Work out the finished part from the listing and answer in its coordinate system (mm). A direction names the side the tool comes from. Coordinates: 2 decimals unless noted, no trailing zeros. Order: outer loops, then holes, each group sorted by start corner. A loop starts at its lowest first (then second) coordinate and runs counter-clockwise, first axis right, second up. Notation, with made-up numbers: (-5.5, -26) -> (22.5, -26) arc R16 cw to (22.5, -8) -> close; hole circle Ø4 at (52.25, -15). An arc over 180 degrees is marked (long way). Write item = value, one per line. Start each with the question number.
Q1. The part is cut by section C-C, the plane y = -8. Determine the outline of the cut face in (x, z), plus the area to 3 significant figures.
Q2. Which of the six approach directions +Z, -Z, +X, -X, +Y, -Y give full straight-line access (tool end or side, diameter ignored) to faces 4 (the flat face through (4, -6, -120)), 5 (the flat face through (3.94, -8.17, 24.15)), 6 (the flat face through (-19, -22, -61))?
Q3. The part is cut by section B-B, the plane x = 2. Determine the outline of the cut face in (y, z), plus the area to 3 significant figures.
Q4. The part is cut by section D-D, the plane z = 22. Determine the outline of the cut face in (x, y), plus the area to 3 significant figures.
Q5. Flat-ended cylindrical pins translate along their axes: pin 1 (1.6 mm diameter, centred on x = -43, y = -13.5, fed in from -Z); pin 2 (1.5 mm diameter, centred on x = -34.5, z = -126, fed in from +Y); pin 3 (8 mm diameter, centred on y = -7, z = -4.5, fed in from +X); pin 4 (1.6 mm diameter, centred on x = -40.5, y = -14, fed in from +Z). Find the tip coordinate at first contact, or state that the pin passes through.
Q6. For a pull along X with two mould halves and no side action, classify faces 1 (the flat face through (-42, -13, -111)), 2 (the flat face through (-38, -16, -59)), 3 (the flat face through (-46, -16, -59)) as +X half, -X half, draft (parallel to the pull), parting line (faces both ways), or undercut.
Q7. The part is cut by section A-A, the plane z = -45. Determine the outline of the cut face in (x, y), plus the area to 3 significant figures.
Q8. Straight lines are drawn through the part: L1, parallel to X at y = -17, z = 8; L2, parallel to Z at x = -14, y = -27; L3, parallel to X at y = -25.25, z = 22. For each, find the intervals that lie inside material, in ascending order. Write a range as from..to.
```python
from build123d import *

# Parameters (mm, degrees)
DODANIE_WYCI_GNI_CIE1_DEPTH = 8
DODANIE_WYCI_GNI_CIE2_REACH = 171.163
SZKIC2_W                    = 200
SZKIC2_H                    = 8
ZAOKR_GLENIE1_R             = 3
ZAOKR_GLENIE2_R             = 3
SZKIC3_R                    = 7.5
WYTNIJ_WYCI_GNI_CIE1_DEPTH  = 170.162643752


with BuildPart() as part:
    # Szkic1 → Dodanie-wyci_gni_cie1 (new body)
    with BuildSketch(Plane(origin=(0, 0, 0), x_dir=(0, 0, -1), z_dir=(1, 0, 0))):
        with BuildLine():
            Line((0, 0), (-8.660254038, 0))
            ThreePointArc((-8.660254038, 0), (-9.954349263, -0.170370869), (-11.160254038, -0.669872981))
            Line((-11.160254038, -0.669872981), (-37.5, -15.877132403))
            ThreePointArc((-37.5, -15.877132403), (-39.330127019, -17.707259422), (-40, -20.207259422))
            Line((-40, -20.207259422), (-40, -30))
            Line((-40, -30), (160, -30))
            Line((160, -30), (160, -20.207259422))
            ThreePointArc((160, -20.207259422), (159.330127019, -17.707259422), (157.5, -15.877132403))
            Line((157.5, -15.877132403), (131.160254038, -0.669872981))
            ThreePointArc((131.160254038, -0.669872981), (129.954349263, -0.170370869), (128.660254038, 0))
            Line((128.660254038, 0), (120, 0))
            Line((120, 0), (120, -13))
            Line((120, -13), (102.3, -13))
            Line((102.3, -13), (102.3, -15))
            Line((102.3, -15), (17.7, -15))
            Line((17.7, -15), (17.7, -13))
            Line((17.7, -13), (0, -13))
            Line((0, -13), (0, 0))
        make_face()
    extrude(amount=DODANIE_WYCI_GNI_CIE1_DEPTH)


with BuildPart() as body_2:
    # Lustro3: mirrored copy
    add(part.part.mirror(Plane.ZY.offset(19)))

    # Szkic2 → Dodanie-wyci_gni_cie2 (add, up to next)
    with BuildSketch(Plane.ZY, mode=Mode.PRIVATE) as dodanie_wyci_gni_cie2_sk1:
        with Locations((-60, -26)):
            Rectangle(SZKIC2_W, SZKIC2_H)
    dodanie_wyci_gni_cie2_tool1 = extrude(dodanie_wyci_gni_cie2_sk1.sketch, amount=DODANIE_WYCI_GNI_CIE2_REACH, mode=Mode.PRIVATE) - body_2.part

    add(part.part)  # Dodanie-wyci_gni_cie2 merges part
    add(dodanie_wyci_gni_cie2_tool1.solids().sort_by_distance((0, -26, -60))[0])

    # Zaokr_glenie1
    zaokr_glenie1_edges = [body_2.edges().sort_by_distance(p)[0] for p in [
        (8, -30, -60),
        (-46, -30, -60),
    ]]
    fillet(zaokr_glenie1_edges, radius=ZAOKR_GLENIE1_R)

    # Zaokr_glenie2
    zaokr_glenie2_edges = [body_2.edges().sort_by_distance(p)[0] for p in [
        (0, -22, -60),
        (-38, -22, -60),
    ]]
    fillet(zaokr_glenie2_edges, radius=ZAOKR_GLENIE2_R)

    # Szkic3 → Wytnij-wyci_gni_cie1 (cut, through all)
    with BuildSketch(Plane.XZ.offset(30)):
        with Locations(Location((-18.58033314, 22, 0), (0, 0, 270))):
            Circle(SZKIC3_R)
        with Locations(Location((-18.58033314, -142, 0), (0, 0, 270))):
            Circle(SZKIC3_R)
    extrude(amount=-WYTNIJ_WYCI_GNI_CIE1_DEPTH, mode=Mode.SUBTRACT)


solid = body_2.part
```
Model answer:
q1.outline = (-46, -143.86) -> (-38, -143.86) -> (-38, -120) -> (-46, -120) -> close; (-46, 0) -> (-38, 0) -> (-38, 23.86) -> (-46, 23.86) -> close; (0, -143.86) -> (8, -143.86) -> (8, -120) -> (0, -120) -> close; (0, 0) -> (8, 0) -> (8, 23.86) -> (0, 23.86) -> close
q1.area = 763 mm2
q2.face_4 = +X, -X, +Y
q2.face_5 = +Z, +X, -X, +Y
q2.face_6 = +Z, -Z, +Y
q3.outline = (-30, -160) -> (-20.21, -160) arc R5 ccw to (-15.88, -157.5) -> (-0.67, -131.16) arc R5 ccw to (0, -128.66) -> (0, -120) -> (-13, -120) -> (-13, -102.3) -> (-15, -102.3) -> (-15, -17.7) -> (-13, -17.7) -> (-13, 0) -> (0, 0) -> (0, 8.66) arc R5 ccw to (-0.67, 11.16) -> (-15.88, 37.5) arc R5 ccw to (-20.21, 40) -> (-30, 40) -> close
q3.area = 3,750 mm2
q4.outline = (-46, -27) arc R3 ccw to (-43, -30) -> (-26.08, -30) -> (-26.08, -22) -> (-35, -22) arc R3 cw to (-38, -19) -> (-38, -6.93) -> (-46, -6.93) -> close; (-11.08, -30) -> (5, -30) arc R3 ccw to (8, -27) -> (8, -6.93) -> (0, -6.93) -> (0, -19) arc R3 cw to (-3, -22) -> (-11.08, -22) -> close
q4.area = 553 mm2
q5.pin_1 = -154.77
q5.pin_2 = -21.99
q5.pin_3 = through
q5.pin_4 = 35.63
q6.face_1 = draft
q6.face_2 = undercut
q6.face_3 = -X half
q7.outline = (-46, -27) arc R3 ccw to (-43, -30) -> (5, -30) arc R3 ccw to (8, -27) -> (8, -15) -> (0, -15) -> (0, -19) arc R3 cw to (-3, -22) -> (-35, -22) arc R3 cw to (-38, -19) -> (-38, -15) -> (-46, -15) -> close
q7.area = 544 mm2
q8.L1 = -46..-38, 0..8
q8.L2 = -160..-147.94, -136.06..16.06, 27.94..40
q8.L3 = -46..-26.08, -11.08..8
